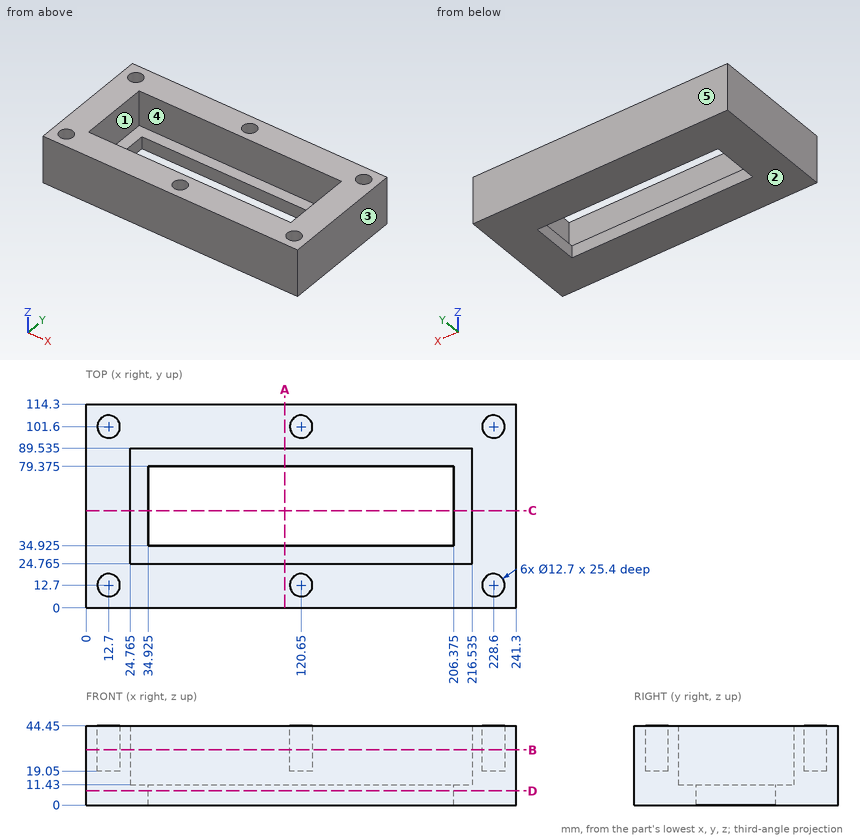
Geometry: see drawing. Coordinates: mm, zero at the bounding-box minimum. A direction names the side the tool comes from. Round coordinates to 2 decimals unless told otherwise and drop trailing zeros. Loops run counter-clockwise (first coordinate to the right, second up) from the corner with the lowest first, then second, coordinate; pieces in that order, holes last. Notation, with made-up numbers: M -30,31.5 L 4,31.5 A25 cw 4,59.5 Z; hole C 89,5.25 d8. An arc over 180 degrees is marked long. Use a Markdown table: item, result. Add a question column.
1. Pull-direction query (X, two-part tool) for the marked faces 3, 4 and 5; classes: +X half, -X half, draft (parallel to the pull), parting line (faces both ways), or undercut.
2. Cut plane D-D, the plane z = 8. Output: boundary loops of the cut face in (x, y) (3 decimals), and give its area (3 significant figures).
3. Cut plane C-C, the plane y = 54.5. Output: boundary loops of the cut face in (x, z) (3 decimals), and give its area (3 significant figures).
4. Contact query for flat-ended pins moving along their axis: pin 1 (3 mm diameter, centred on y = 77.5, z = 40, fed in from -X); pin 2 (6.5 mm diameter, centred on x = 11.5, y = 11.5, fed in from +Z). Output: stop coordinate, or through.
5. Cut plane B-B, the plane z = 31. Output: boundary loops of the cut face in (x, y) (3 decimals), and give its area (3 significant figures).
6. Ray query, line 1 along X through (y, z) = (101, 35); line 2 along Y through (x, z) = (120.65, 30) (3 decimals); line 3 along Y through (x, z) = (228.6, 38.75). Return the intervals inside material, ascending. Write a range as [from, to].
7. Set-up query: the marked faces 1 and 2. Return all of +Z, -Z, +X, -X, +Y, -Y with unobstructed straight access to the full face (end or side cutting, diameter ignored); none if empty.
8. Cut plane A-A, the plane x = 111.5. Output: boundary loops of the cut face in (y, z) (3 decimals).
Solution:
| question | item | result |
|---|---|---|
| 1 | face 3 | +X half |
| 1 | face 4 | undercut |
| 1 | face 5 | draft |
| 2 | outline | M 0,0 L 241.3,0 L 241.3,114.3 L 0,114.3 Z; hole M 34.925,34.925 L 206.375,34.925 L 206.375,79.375 L 34.925,79.375 Z |
| 2 | area | 20,000 mm2 |
| 3 | outline | M 0,0 L 34.925,0 L 34.925,11.43 L 24.765,11.43 L 24.765,44.45 L 0,44.45 Z; M 206.375,0 L 241.3,0 L 241.3,44.45 L 216.535,44.45 L 216.535,11.43 L 206.375,11.43 Z |
| 3 | area | 2,430 mm2 |
| 4 | pin 1 | stops at x = 0 |
| 4 | pin 2 | stops at z = 19.05 |
| 5 | outline | M 0,0 L 241.3,0 L 241.3,114.3 L 0,114.3 Z; hole C 12.7,12.7 d12.7; hole C 12.7,101.6 d12.7; hole M 24.765,24.765 L 216.535,24.765 L 216.535,89.535 L 24.765,89.535 Z; hole C 120.65,12.7 d12.7; hole C 120.65,101.6 d12.7; hole C 228.6,12.7 d12.7; hole C 228.6,101.6 d12.7 |
| 5 | area | 14,400 mm2 |
| 6 | line 1 | x = [0, 6.38], [19.02, 114.33], [126.97, 222.28], [234.92, 241.3] |
| 6 | line 2 | y = [0, 6.35], [19.05, 24.765], [89.535, 95.25], [107.95, 114.3] |
| 6 | line 3 | y = [0, 6.35], [19.05, 95.25], [107.95, 114.3] |
| 7 | face 1 | +Z |
| 7 | face 2 | -Z, +X, -X, +Y, -Y |
| 8 | outline | M 0,0 L 34.925,0 L 34.925,11.43 L 24.765,11.43 L 24.765,44.45 L 0,44.45 Z; M 79.375,0 L 114.3,0 L 114.3,44.45 L 89.535,44.45 L 89.535,11.43 L 79.375,11.43 Z |
